Input: part model. Units: mm. Frame: model coordinates. Coordinates: 2 decimals unless noted, no trailing zeros. Write each loop counter-clockwise with the first axis right and the second up, starting at its lowest first coordinate (ties: lowest second). Pieces come first, ordered by that corner, then holes. Notation, with made-up numbers: (-20.5, 73.5) - (-12.5, 73.5) arc R10 ccw to (-12.5, 92.5) - close; hole circle Ø6 at (-32, 32). An arc over 180 degrees is marked (long way). Put each result on its own line as item: value. Start each with the question number.
1. Pull-direction query (Y, two-part tool) for faces 1 (the flat face through (-3, 38.1, -1)), 2 (the flat face through (-3, 1, 38.1)), 3 (the cylindrical face through (-3.219, -11.795, 18.085)); classes: released by +Y, released by -Y, zero draft, split by the parting line, or undercut.
2. Cut plane D-D, the plane x = -2.75. Return loops of the section in (y, z), and give its area (3 significant figures).
3. Cut plane A-A, the plane z = 0. Return loops of the section in (x, y), and give its area (3 significant figures).
4. Cut plane C-C, the plane y = 13.5. Return loops of the section in (x, z), and give its area (3 significant figures).
5. Cut plane B-B, the plane y = 0. Return loops of the section in (x, z), and give its area (3 significant figures).
6. Line query: line 1 (Y direction, x = -1.25, z = 1.5); line 2 (Y direction, x = -3.75, z = 0); line 3 (Y direction, x = -1.5, z = -20.5). Output: solid intervals per line, ascending.
Autodesk Inventor part; units mm, degrees
ref_plane "YZ Plane" through (0, 0, 0) normal (1, 0, 0) x (0, 1, 0)
ref_plane "XZ Plane" through (0, 0, 0) normal (0, 1, 0) x (-1, 0, 0)
ref_plane "XY Plane" through (0, 0, 0) normal (0, 0, 1) x (1, 0, 0)
sketch "Sketch1" plane through (0, 0, 0) normal (1, 0, 0) x (0, 1, 0)
  line L0 (-38.1, 38.1) -> (-38.1, -38.1)
  line L1 (-38.1, -38.1) -> (38.1, -38.1)
  line L2 (38.1, -38.1) -> (38.1, 38.1)
  line L3 (38.1, 38.1) -> (-38.1, 38.1)
  line L4 (-38.1, 38.1) -> (38.1, -38.1) construction
  line L5 (-38.1, -38.1) -> (38.1, 38.1) construction
  point P0 (0, 0)
  dimension "d0" = 76.2
  dimension "d1" = 76.2
extrude "Extrusion1" add sketch "Sketch1" against normal blind 6.35
sketch "Sketch4" plane through (-6.35, 0, 0) normal (-1, 0, 0) x (0, 0, 1)
  circle A0 centre (0, -23.8125) radius 2.54
  circle A1 centre (20.6222, -11.9063) radius 2.54
  circle A2 centre (20.6222, 11.9062) radius 2.54
  circle A3 centre (0, 23.8125) radius 2.54
  circle A4 centre (-20.6222, 11.9063) radius 2.54
  circle A5 centre (-20.6222, -11.9062) radius 2.54
  point P0 (0, 0)
  dimension "d13" = 5.08
  dimension "d14" = 23.8125
  dimension "d17" = 360
extrude "Extrusion3" cut sketch "Sketch4" against normal through all
sketch "Sketch5" plane through (-6.35, 0, 0) normal (-1, 0, 0) x (0, 0, 1)
  circle A0 centre (0, 0) radius 5
  dimension "d21" = 10
extrude "Extrusion4" cut sketch "Sketch5" against normal through all
equation "\"d13\" = amHubBoltDiam"
equation "\"d21\" = centerHoleDiam"
equation "\"amHubBoltHoleDiam\" = 47.625"
equation "\"amHubBoltDiam\" = 5.08"
equation "\"centerHoleDiam\" = 10"
properties part number "PlateForConnectionToArm" material "Aluminum 6061"
Report:
1. face 1: released by +Y
1. face 2: zero draft
1. face 3: undercut
2. outline: (-38.1, -38.1) - (38.1, -38.1) - (38.1, 38.1) - (-38.1, 38.1) - close; hole circle Ø5.08 at (-23.81, 0); hole circle Ø5.08 at (-11.91, -20.62); hole circle Ø5.08 at (-11.91, 20.62); hole circle Ø10 at (0, 0); hole circle Ø5.08 at (11.91, -20.62); hole circle Ø5.08 at (11.91, 20.62); hole circle Ø5.08 at (23.81, 0)
2. area: 5,610 mm^2
3. outline: (-6.35, -38.1) - (0, -38.1) - (0, -26.35) - (-6.35, -26.35) - close; (-6.35, -21.27) - (0, -21.27) - (0, -5) - (-6.35, -5) - close; (-6.35, 5) - (0, 5) - (0, 21.27) - (-6.35, 21.27) - close; (-6.35, 26.35) - (0, 26.35) - (0, 38.1) - (-6.35, 38.1) - close
3. area: 356 mm^2
4. outline: (-6.35, -38.1) - (0, -38.1) - (0, -22.6) - (-6.35, -22.6) - close; (-6.35, -18.64) - (0, -18.64) - (0, 18.64) - (-6.35, 18.64) - close; (-6.35, 22.6) - (0, 22.6) - (0, 38.1) - (-6.35, 38.1) - close
4. area: 434 mm^2
5. outline: (-6.35, -38.1) - (0, -38.1) - (0, -5) - (-6.35, -5) - close; (-6.35, 5) - (0, 5) - (0, 38.1) - (-6.35, 38.1) - close
5. area: 420 mm^2
6. line 1: y = -38.1 to -25.86, -21.76 to -4.77, 4.77 to 21.76, 25.86 to 38.1
6. line 2: y = -38.1 to -26.35, -21.27 to -5, 5 to 21.27, 26.35 to 38.1
6. line 3: y = -38.1 to -14.44, -9.37 to 9.37, 14.44 to 38.1
